Can you work these out from the model? Positions are in its coordinate system, mm. A direction names the side the tool comes from. Give positions to 0.01 mm unless a question says otherwise; leave off trailing zeros. Loops run counter-clockwise (first coordinate to the right, second up) from the corner with the lowest first, then second, coordinate; pieces in that order, holes last. Notation, with made-up numbers: (62, 40.25) - (107, 40.25) arc R23 cw to (107, 54.25) - close; hole circle Ø2 at (77.25, 3). An arc over 180 degrees is marked (long way). Answer in a Markdown table with one row per item.
from build123d import *

# Parameters (mm, degrees)
SKETCH1_W           = 110.510118672
SKETCH1_H           = 27.56100364
BOSS_EXTRUDE1_DEPTH = 10


with BuildPart() as part:
    # Sketch1 → Boss-Extrude1 (new body)
    with BuildSketch(Plane.XY):
        with Locations((55.255059336, 13.78050182)):
            Rectangle(SKETCH1_W, SKETCH1_H)
        with BuildLine():
            Line((15.435752348, 18.78050182), (95.074366324, 18.78050182))
            ThreePointArc((95.074366324, 18.78050182), (100.074366324, 13.78050182), (95.074366324, 8.78050182))
            Line((95.074366324, 8.78050182), (15.435752348, 8.78050182))
            ThreePointArc((15.435752348, 8.78050182), (10.435752348, 13.78050182), (15.435752348, 18.78050182))
        make_face(mode=Mode.SUBTRACT)
    extrude(amount=BOSS_EXTRUDE1_DEPTH)


solid = part.part
Q1. Imagine slicing it at A-A, the plane x = 55. Write out the boundary of the cut face in (y, z).
Checked values:
| item | result |
|---|---|
| outline | (0, 0) - (8.78, 0) - (8.78, 10) - (0, 10) - close; (18.78, 0) - (27.56, 0) - (27.56, 10) - (18.78, 10) - close |
Q2. Imagine slicing it at B-B, the plane z = 7.5. Write out the boundary of the cut face in (x, y), and give its area (3 significant figures).
Checked values:
| item | result |
|---|---|
| outline | (0, 0) - (110.51, 0) - (110.51, 27.56) - (0, 27.56) - close; hole (15.44, 8.78) - (95.07, 8.78) arc R5 ccw to (95.07, 18.78) - (15.44, 18.78) arc R5 ccw to start |
| area | 2,170 mm² |
Q3. If I drill on line 1 (Y direction, x = 51.5, z = 1.5); line 2 (X direction, y = 9.25, z = 8.25); line 3 (X direction, y = 13.25, z = 3.5), over which ranges is the centre line in solid material (lowest first)? Write a range as [from, to].
Checked values:
| item | result |
|---|---|
| line 1 | y = [0, 8.78], [18.78, 27.56] |
| line 2 | x = [0, 13.32], [97.19, 110.51] |
| line 3 | x = [0, 10.46], [100.05, 110.51] |
Q4. On a 3-axis mill with a long thin cutter (end or side, diameter ignored), from which of +Z, -Z, +X, -X, +Y, -Y can I reach the whole of each face in a straight line? I mean faces 1 (the face through (54, 8, 10)), 2 (the face through (56, 8.781, 5)). Say none if no direction works.
Checked values:
| item | result |
|---|---|
| face 1 | +Z, +X, -X, +Y, -Y |
| face 2 | +Z, -Z |
Q5. Imagine slicing it at C-C, the plane y = 17. Write out the boundary of the cut face in (x, z), and give its area (3 significant figures).
Checked values:
| item | result |
|---|---|
| outline | (0, 0) - (11.61, 0) - (11.61, 10) - (0, 10) - close; (98.9, 0) - (110.51, 0) - (110.51, 10) - (98.9, 10) - close |
| area | 232 mm² |
Q6. If we mould it in two halves opening along X, with no side actions, what happens to faces 3 (the face through (55, 18.781, 5)), 4 (the face through (110.51, 14, 5)), 5 (the face through (100.073, 13.89, 4.93)), 6 (the face through (54, 27.561, 5))? For each: released by +X, released by -X, zero draft, split by the parting line, or undercut.
Checked values:
| item | result |
|---|---|
| face 3 | undercut |
| face 4 | released by +X |
| face 5 | undercut |
| face 6 | zero draft |
